Here's how the part is built. I have some questions about the finished solid (model axes, mm). Face numbers are marked on the shaded views. A direction names the side the tool comes from. Coordinates: 2 decimals unless noted, no trailing zeros. Write each loop counter-clockwise with the first axis right and the second up, starting at its lowest first coordinate (ties: lowest second). Pieces come first, ordered by that corner, then holes.
Item 1: I want a section at D-D (y = -10). Please give me the cut outline in (x, z).
Item 2: For the marked faces 4 and 5, which set-ups out of +Z, -Z, +X, -X, +Y, -Y let a thin tool reach every point of the face, with its end or its side?
Item 3: If we mould it in two halves opening along Y, with no side actions, what happens to the marked faces 1, 2 and 3? For each: pulls with the +Y half, pulls with the -Y half, needs draft (parallel to the pull), parting line crosses it, or undercut.
Item 4: I want a section at A-A (x = 0). Please give me the cut outline in (y, z), and give its area (3 significant figures).
Item 5: I want a section at B-B (z = 16.5). Count the separate pieces of the cut face and the enclosed holes in it, and give its area (3 significant figures).
Item 6: I want a section at C-C (x = -32). Please give me the cut outline in (y, z), and give its area (3 significant figures).
Item 7: Please list where these lines run through material, in increasing order: line 1 (Y direction, x = 0, z = 14.5); line 2 (X direction, y = 10, z = 13); line 3 (X direction, y = 9.5, z = 16).
Item 8: I'm going to push flat-ended pins straight in: P1, Ø8.5, axis at x = 35.96, y = 11.68, coming from the +Z side; P2, Ø10, axis at x = -1.5, z = 25, coming from the +Y side; P3, Ø5, axis at x = -9.5, z = 5, coming from the -Y side; P4, Ø5, axis at y = -16.5, z = 10.5, coming from the -X side. Where does each tip first touch, or does it pass through?
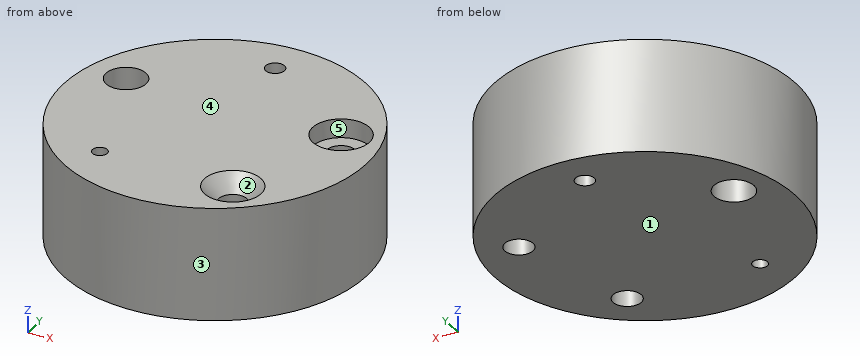
Autodesk Inventor part; units mm, degrees
ref_plane "YZ Plane" through (0, 0, 0) normal (1, 0, 0) x (0, 1, 0)
ref_plane "XZ Plane" through (0, 0, 0) normal (0, 1, 0) x (-1, 0, 0)
ref_plane "XY Plane" through (0, 0, 0) normal (0, 0, 1) x (1, 0, 0)
sketch "Sketch1" plane through (0, 0, 0) normal (0, 0, 1) x (1, 0, 0)
  circle A0 centre (0, 0) radius 50.8
  dimension "d0" = 101.6
extrude "Extrusion1" add sketch "Sketch1" along normal blind 38.1
sketch "Sketch2" plane through (0, 0, 38.1) normal (0, 0, 1) x (1, 0, 0)
  circle A0 centre (0, 0) radius 50.8
  point P0 (0, 37.809)
  point P1 (-35.9585, 11.6836)
  point P2 (-22.2236, -30.5881)
  point P3 (22.2236, -30.5881)
  point P4 (35.9585, 11.6836)
  dimension "d5" = 360
hole "Hole1" at (0, 37.809, 38.1) direction (0, 0, -1) diameter 6.35 end through all
hole "Hole2" at (35.9585, 11.6836, 38.1) direction (0, 0, -1) diameter 9.525 end through all counterbore diameter 19.05 counterbore depth 6.35
hole "Hole3" at (22.2236, -30.5881, 38.1) direction (0, 0, -1) diameter 9.525 end through all countersink diameter 19.05 countersink angle 82
hole "Hole4" at (-22.2236, -30.5881, 38.1) direction (0, 0, -1) diameter 4.9784 end through all
hole "Hole5" at (-35.9585, 11.6836, 38.1) direction (0, 0, -1) diameter 13.4874 end through all
properties part number "CircularPlate"
Answer:
1. outline: (-49.81, 0) - (49.81, 0) - (49.81, 38.1) - (-49.81, 38.1) - close
2. face 4: +Z, +X, -X, +Y, -Y
2. face 5: +Z
3. face 1: needs draft
3. face 2: undercut
3. face 3: parting line crosses it
4. outline: (-50.8, 0) - (34.63, 0) - (34.63, 38.1) - (-50.8, 38.1) - close; (40.98, 0) - (50.8, 0) - (50.8, 38.1) - (40.98, 38.1) - close
4. area: 3,630 mm2
5. separate pieces: 1
5. enclosed holes: 5
5. area: 7,770 mm2
6. outline: (-39.45, 0) - (6.22, 0) - (6.22, 38.1) - (-39.45, 38.1) - close; (17.14, 0) - (39.45, 0) - (39.45, 38.1) - (17.14, 38.1) - close
6. area: 2,590 mm2
7. line 1: y = -50.8 to 34.63, 40.98 to 50.8
7. line 2: x = -49.81 to -42.49, -29.43 to 31.5, 40.41 to 49.81
7. line 3: x = -49.9 to -42.34, -29.58 to 31.73, 40.19 to 49.9
8. P1: passes through
8. P2: stops at y = 50.8
8. P3: stops at y = -50.32
8. P4: stops at x = -48.83
